from build123d import *

# Parameters (mm, degrees)
BOSS_EXTRUDE1_DEPTH = 0.635
FILLET1_R           = 9.525
SKETCH2_R           = 25.4
SKETCH2_R_2         = 6.35
SKETCH2_W           = 25.4
SKETCH2_H           = 25.4
SKETCH2_W_2         = 63.5
SKETCH2_H_2         = 47.625
SKETCH2_W_3         = 28.575
CUT_EXTRUDE1_DEPTH  = 390.952780599


with BuildPart() as part:
    # Sketch1 → Boss-Extrude1 (new body)
    with BuildSketch(Plane(origin=(0, 0, 0), x_dir=(1, 0, 0), z_dir=(0, 1, 0))):
        with BuildLine():
            Line((-289.73775964, -52.172972973), (-289.73775964, 151.027027027))
            Line((-289.73775964, 151.027027027), (119.83724036, 151.027027027))
            ThreePointArc((119.83724036, 151.027027027), (141.932070827, 146.12872104), (159.886674172, 132.351669336))
            Line((159.886674172, 132.351669336), (363.971740247, -110.867441355))
            Line((363.971740247, -110.867441355), (306.753969954, -150.931755434))
            Line((306.753969954, -150.931755434), (65.86224036, -52.172972973))
            Line((65.86224036, -52.172972973), (-289.73775964, -52.172972973))
        make_face()
    extrude(amount=BOSS_EXTRUDE1_DEPTH)

    # Fillet1
    fillet1_edges = [part.edges().sort_by_distance(p)[0] for p in [
        (-289.73775964, 0.3175, 52.172972973),
        (-289.73775964, 0.3175, -151.027027027),
        (363.971740247, 0.3175, 110.867441355),
        (306.753969954, 0.3175, 150.931755434),
    ]]
    fillet(fillet1_edges, radius=FILLET1_R)

    # Sketch2 → Cut-Extrude1 (cut, through all)
    with BuildSketch(Plane(origin=(0, 0.635, 0), x_dir=(1, 0, 0), z_dir=(0, 1, 0))):
        with Locations(Location((-169.08775964, -1.372972973, 0), (0, 0, 270))):
            Circle(SKETCH2_R)
        with Locations(Location((-226.23775964, 74.827027027, 0), (0, 0, 270))):
            Circle(SKETCH2_R_2)
        with BuildLine():
            Line((232.109731363, 31.667957705), (232.109731363, -44.532042295))
            Line((232.109731363, -44.532042295), (308.309731363, -44.532042295))
            Line((308.309731363, -44.532042295), (228.651141857, 50.401367929))
            ThreePointArc((228.651141857, 50.401367929), (231.237839047, 41.192957705), (232.109731363, 31.667957705))
        make_face()
        Polygon((-121.46275964, -52.172972973), (-121.46275964, -26.772972973), (-64.31275964, -26.772972973), (-45.26275964, -20.422972973), (-7.16275964, -20.422972973), (-7.16275964, -52.172972973), align=None)
        with Locations((-213.53775964, 112.927027027)):
            Rectangle(SKETCH2_W, SKETCH2_H)
        with Locations((30.93724036, 109.752027027)):
            Rectangle(SKETCH2_W_2, SKETCH2_H)
        with Locations((65.86224036, -33.567113065)):
            Rectangle(SKETCH2_W, SKETCH2_H_2)
        with Locations((-205.60025964, -39.472972973)):
            Rectangle(SKETCH2_W_3, SKETCH2_H)
    extrude(amount=-CUT_EXTRUDE1_DEPTH, mode=Mode.SUBTRACT)


solid = part.part
Geometry check sheet. Reference: the model listing, model coordinates, mm. Give positions to 0.01 mm unless a question says otherwise; leave off trailing zeros. Loops run counter-clockwise (first coordinate to the right, second up) from the corner with the lowest first, then second, coordinate; pieces in that order, holes last. Notation, with made-up numbers: M 58,67 L 80,67 A37 ccw 80,104 Z; hole C -11,-12.75 d3. An arc over 180 degrees is marked long. Answer as a JSON object with one key per item and string values. Group by question number.
Item 1: Sectioned sample at D-D on z = -109.5. Record the boundary of the cut face in (x, y) (1 decimal).
Item 2: Mould release check, pull along Z, two halves, no side actions. Record for faces 1 (the flat face through (333.55, 0.31, 132.17)), 2 (the flat face through (39, 0, -36)), 3 (the cylindrical face through (-191.622, 0.322, 13.094)), 4 (the cylindrical face through (141.642, 0.313, -146.263)): pulls with the +Z half, pulls with the -Z half, needs draft (parallel to the pull), parting line crosses it, or undercut.
Item 3: Material ranges on L1, parallel to Z at x = -223.5, y = 0.25; L2, parallel to X at y = 0.3, z = -114.5; L3, parallel to Z at x = -82, y = 0.35, recorded low to high.
Item 4: Sectioned sample at B-B on z = -17. Record the boundary of the cut face in (x, y) (3 decimals), plus the area to 3 significant figures.
Item 5: Sectioned sample at A-A on z = 34. Record the boundary of the cut face in (x, y) (3 decimals), plus the area to 3 significant figures.
Item 6: Sectioned sample at C-C on x = -156. Record the boundary of the cut face in (y, z) (3 decimals), plus the area to 3 significant figures.
Findings below:
{
 "1": {"outline": "M -289.7,0 L -226.2,0 L -226.2,0.6 L -289.7,0.6 Z; M -200.8,0 L -0.8,0 L -0.8,0.6 L -200.8,0.6 Z; M 62.7,0 L 179.1,0 L 179.1,0.6 L 62.7,0.6 Z"},
 "2": {"face 1": "pulls with the +Z half", "face 2": "needs draft", "face 3": "undercut", "face 4": "pulls with the -Z half"},
 "3": {"L1": "-151.03 to -125.63, -100.23 to -80.56, -69.1 to 52.17", "L2": "-289.74 to -226.24, -200.84 to -0.81, 62.69 to 174.87", "L3": "-151.03 to 26.77"},
 "4": {"outline": "M -289.738,0 L -186.626,0 L -186.626,0.635 L -289.738,0.635 Z; M -151.549,0 L 232.11,0 L 232.11,0.635 L -151.549,0.635 Z", "area": "309 mm2"},
 "5": {"outline": "M -289.738,0 L -219.888,0 L -219.888,0.635 L -289.738,0.635 Z; M -191.313,0 L -121.463,0 L -121.463,0.635 L -191.313,0.635 Z; M -7.163,0 L 53.162,0 L 53.162,0.635 L -7.163,0.635 Z; M 78.562,0 L 232.11,0 L 232.11,0.635 L 78.562,0.635 Z", "area": "225 mm2"},
 "6": {"outline": "M 0,-151.027 L 0.635,-151.027 L 0.635,-20.396 L 0,-20.396 Z; M 0,23.142 L 0.635,23.142 L 0.635,52.173 L 0,52.173 Z", "area": "101 mm2"}
}
